The listing builds one solid part. Answer for the finished solid, in the listing's coordinates (mm). A direction names the side the tool comes from. Give positions to 0.01 mm unless a question says otherwise; leave off trailing zeros. Order: outer loops, then holes, each group sorted by start corner. A loop starts at its lowest first (then second) coordinate and runs counter-clockwise, first axis right, second up. Notation, with made-up numbers: M 27,84.5 L 67,84.5 A27 cw 67,119.5 Z; hole C 0,29.25 d2. An arc over 180 degrees is marked long. Answer as a JSON object with one key per item and string values. Group by question number.
```python
from build123d import *

# Parameters (mm, degrees)
F1_DEPTH = 2
F2_R     = 5
F4_DEPTH = 2


# Not quite as in the source:
# - a feature names something its author has since deleted; it is built from what else it names


with BuildPart() as f1:
    # F0 (on Front) → F1 (new body)
    with BuildSketch(Plane.XZ):
        with BuildLine():
            Line((0, 5.5), (0, 0))
            Line((0, 0), (40, 0))
            Line((40, 0), (40, 5.5))
            Line((40, 5.5), (31, 5.5))
            ThreePointArc((31, 5.5), (28, 2.5), (25, 5.5))
            Line((25, 5.5), (0, 5.5))
        make_face()
        with BuildLine():
            Line((40, 5.5), (40, 0))
            Line((40, 0), (40, -2.5))
            ThreePointArc((40, -2.5), (41.05572809, 1.972135955), (44, 5.5))
            Line((44, 5.5), (40, 5.5))
        make_face()
        with BuildLine():
            Line((0, 11), (0, 5.5))
            Line((0, 5.5), (25, 5.5))
            ThreePointArc((25, 5.5), (28, 8.5), (31, 5.5))
            Line((31, 5.5), (40, 5.5))
            Line((40, 5.5), (40, 11))
            Line((40, 11), (0, 11))
        make_face()
        with BuildLine():
            Line((40, 11), (40, 5.5))
            Line((40, 5.5), (44, 5.5))
            ThreePointArc((44, 5.5), (41.05572809, 9.027864045), (40, 13.5))
            Line((40, 13.5), (40, 11))
        make_face()
        with BuildLine():
            Line((45, -2.5), (40, -2.5))
            ThreePointArc((40, -2.5), (50, -12.5), (60, -2.5))
            ThreePointArc((60, -2.5), (58.94427191, 1.972135955), (56, 5.5))
            ThreePointArc((56, 5.5), (53.1622776602, 4.0131670195), (50, 3.5))
            Line((50, 3.5), (50, 2.5))
            ThreePointArc((50, 2.5), (53.5355339059, 1.0355339059), (55, -2.5))
            ThreePointArc((55, -2.5), (50, -7.5), (45, -2.5))
        make_face()
        with BuildLine():
            ThreePointArc((44, 5.5), (41.05572809, 1.972135955), (40, -2.5))
            Line((40, -2.5), (45, -2.5))
            ThreePointArc((45, -2.5), (46.4644660941, 1.0355339059), (50, 2.5))
            Line((50, 2.5), (50, 3.5))
            ThreePointArc((50, 3.5), (46.8377223398, 4.0131670195), (44, 5.5))
        make_face()
        with BuildLine():
            ThreePointArc((40, 13.5), (41.05572809, 9.027864045), (44, 5.5))
            ThreePointArc((44, 5.5), (46.8377223398, 6.9868329805), (50, 7.5))
            Line((50, 7.5), (50, 8.5))
            ThreePointArc((50, 8.5), (46.4644660941, 9.9644660941), (45, 13.5))
            Line((45, 13.5), (40, 13.5))
        make_face()
        with BuildLine():
            Line((50, 5.5), (44, 5.5))
            ThreePointArc((44, 5.5), (46.8377223398, 4.0131670195), (50, 3.5))
            Line((50, 3.5), (50, 5.5))
        make_face()
        with BuildLine():
            ThreePointArc((50, 7.5), (46.8377223398, 6.9868329805), (44, 5.5))
            Line((44, 5.5), (50, 5.5))
            Line((50, 5.5), (50, 7.5))
        make_face()
        with BuildLine():
            ThreePointArc((60, 13.5), (50, 23.5), (40, 13.5))
            Line((40, 13.5), (45, 13.5))
            ThreePointArc((45, 13.5), (50, 18.5), (55, 13.5))
            ThreePointArc((55, 13.5), (53.5355339059, 9.9644660941), (50, 8.5))
            Line((50, 8.5), (50, 7.5))
            ThreePointArc((50, 7.5), (53.1622776602, 6.9868329805), (56, 5.5))
            ThreePointArc((56, 5.5), (58.94427191, 9.027864045), (60, 13.5))
        make_face()
        with BuildLine():
            ThreePointArc((56, 5.5), (53.1622776602, 6.9868329805), (50, 7.5))
            Line((50, 7.5), (50, 5.5))
            Line((50, 5.5), (56, 5.5))
        make_face()
        with BuildLine():
            Line((50, 5.5), (50, 3.5))
            ThreePointArc((50, 3.5), (53.1622776602, 4.0131670195), (56, 5.5))
            Line((56, 5.5), (50, 5.5))
        make_face()
    extrude(amount=F1_DEPTH)

    # F2
    f2_edges = [f1.edges().sort_by_distance(p)[0] for p in [
        (40, -1, 11),
        (40, -1, 0),
        (0, -1, 11),
        (0, -1, 0),
    ]]
    fillet(f2_edges, radius=F2_R)

    # F3 (on face) → F4 (cut, through all)
    with BuildSketch(Plane.XZ.offset(2)):
        with BuildLine():
            Line((25.0419601085, 6), (0, 6))
            Line((0, 6), (0, 5))
            Line((0, 5), (25.0419601085, 5))
            ThreePointArc((25.0419601085, 5), (25, 5.5), (25.0419601085, 6))
        make_face()
        with BuildLine():
            Line((34, 6), (30.9580398915, 6))
            ThreePointArc((30.9580398915, 6), (30.9894915684, 5.7508787808), (31, 5.5))
            ThreePointArc((31, 5.5), (30.9894915684, 5.2491212192), (30.9580398915, 5))
            Line((30.9580398915, 5), (34, 5))
            Line((34, 5), (34, 6))
        make_face()
    extrude(amount=-F4_DEPTH, mode=Mode.SUBTRACT)


solid = f1.part
```
Item 1: Section D-D (z = 19.5) is taken. Determine the outline of the cut face in (x, y), and give its area (3 significant figures).
Item 2: Section A-A (x = 10.5) is taken. Determine the outline of the cut face in (y, z).
Item 3: Consider probe 1 along Z at (x, y) = (23.5, -1); probe 2 along Z at (x, y) = (51.5, -1.85); probe 3 along X at (y, z) = (-0.25, -5.5). Determine where each line is inside the solid, lowest interval first. Write a range as from..to.
Item 4: Section C-C (y = -1.55) is taken. Count the separate pieces of the cut face and the enclosed holes in it, and give its area (3 significant figures).
Item 5: Determine the mould class of faces 1 (the flat face through (13, -1, 6)), 2 (the flat face through (20, -1, 0)), 3 (the flat face through (36, 0, 6)) for opening direction Z: released by +Z, released by -Z, zero draft, split by the parting line, or undercut.
Item 6: A tool of negligible diameter and unlimited length cuts with its end or side. For faces 4 (the cylindrical face through (1, -1, 2)), 5 (the cylindrical face through (27.9, -1, 8.5)), 6 (the flat face through (32, -1, 5)), 7 (the flat face through (20, -1, 11)), from which of +Z, -Z, +X, -X, +Y, -Y can it reach the whole face along a straight path? Write none if from no direction.
Item 7: Flat-ended cylindrical pins translate along their axes: P1, Ø0.6, axis at x = 32, y = -1, coming from the +Z side; P2, Ø0.6, axis at x = 15, y = -0.5, coming from the -Z side. Find the tip coordinate at first contact, or state that the pin passes through.
Item 8: Section B-B (z = 4) is taken. Determine the outline of the cut face in (x, y).
Values found:
{
 "1": {"outline": "M 42,-2 L 58,-2 L 58,0 L 42,0 Z", "area": "32.0 mm^2"},
 "2": {"outline": "M -2,0 L 0,0 L 0,5 L -2,5 Z; M -2,6 L 0,6 L 0,11 L -2,11 Z"},
 "3": {"probe 1": "z = 0..5, 6..11", "probe 2": "z = -12.39..-7.27, 2.27..8.73, 18.27..23.39", "probe 3": "x = 40.46..46, 54..59.54"},
 "4": {"separate pieces": "1", "enclosed holes": "2", "area": "840 mm^2"},
 "5": {"face 1": "undercut", "face 2": "released by -Z", "face 3": "zero draft"},
 "6": {"face 4": "-Z, -X, +Y, -Y", "face 5": "+Y, -Y", "face 6": "-X, +Y, -Y", "face 7": "+Z, -X, +Y, -Y"},
 "7": {"P1": "stops at z = 11", "P2": "stops at z = 0"},
 "8": {"outline": "M 0.1,-2 L 25.4,-2 L 25.4,0 L 0.1,0 Z; M 30.6,-2 L 57.6,-2 L 57.6,0 L 30.6,0 Z"}
}
